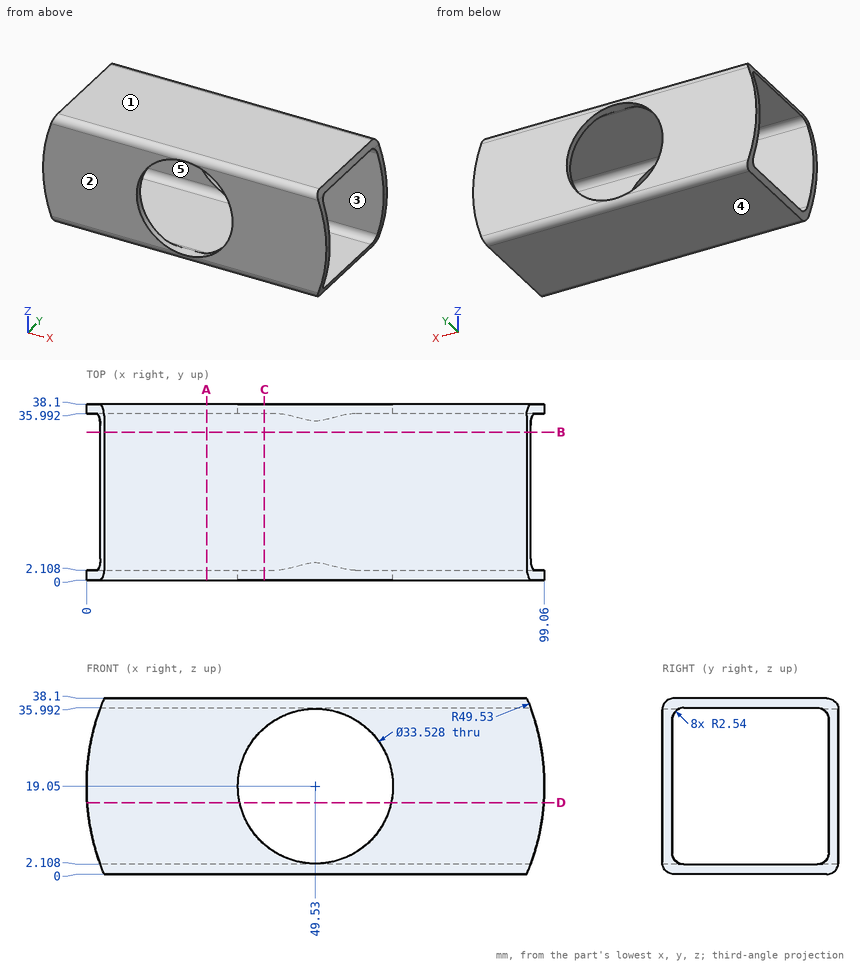
The drawing under review shows one solid part. Ordinate dimensions are in mm from its lowest x, y, z. A direction names the side the tool comes from. Give positions to 0.01 mm unless a question says otherwise; leave off trailing zeros. Write each loop counter-clockwise with the first axis right and the second up, starting at its lowest first coordinate (ties: lowest second). Pieces come first, ordered by that corner, then holes. Notation, with made-up numbers: M 83.5,57 L 125.5,57 A38 ccw 125.5,96 Z; hole C -34.75,69.25 d4. An arc over 180 degrees is marked long. Write each question's results on one line, items separated by ' | '. Start each with the question number.
1. We need section A-A (x = 26). Write out the cut boundary in (y, z).
2. Mouldability with a two-part tool opening along Y and no side actions: class the marked faces 1, 2 and 3 as released by +Y, released by -Y, zero draft, split by the parting line, or undercut.
3. We need section D-D (z = 15.5). Write out the cut boundary in (x, y).
4. For probe 1 along Y at (x, z) = (9, 7); probe 2 along Z at (x, y) = (49.53, 35.85), list the stretches that pass through material, from the lowest coordinate up. Write a range as [from, to].
5. For the marked faces 4 and 5, list the 3-axis set-ups (+Z, -Z, +X, -X, +Y, -Y) from which the entire face can be reached by the end or side of a thin tool; tool diameter is ignored.
6. We need section C-C (x = 38.5). Write out the cut boundary in (y, z), and give its area (3 significant figures).
7. We need section B-B (y = 32). Write out the cut boundary in (x, z), and give its area (3 significant figures).
8. Insertion check: pin 1 Ø12 at (y, z) = (34, 18.5) entering from -X. The pin has a flat end and moves straight along its axis. Give the tip position at first contact, or say it passes through.
Results found:
1) outline: M 0,2.54 A2.54 ccw 2.54,0 L 35.56,0 A2.54 ccw 38.1,2.54 L 38.1,35.56 A2.54 ccw 35.56,38.1 L 2.54,38.1 A2.54 ccw 0,35.56 Z; hole M 2.11,4.65 A2.54 ccw 4.65,2.11 L 33.45,2.11 A2.54 ccw 35.99,4.65 L 35.99,33.45 A2.54 ccw 33.45,35.99 L 4.65,35.99 A2.54 ccw 2.11,33.45 Z
2) face 1: zero draft | face 2: released by -Y | face 3: undercut
3) outline: M 0.13,0 L 33.15,0 L 33.15,2.11 L 0.13,2.11 Z; M 0.13,35.99 L 33.15,35.99 L 33.15,38.1 L 0.13,38.1 Z; M 65.91,0 L 98.93,0 L 98.93,2.11 L 65.91,2.11 Z; M 65.91,35.99 L 98.93,35.99 L 98.93,38.1 L 65.91,38.1 Z
4) probe 1: y = [0, 2.11], [35.99, 38.1] | probe 2: z = [0.02, 2.29], [35.81, 38.08]
5) face 4: -Z, +X, -X, +Y, -Y | face 5: +X, -X
6) outline: M 0,2.54 A2.54 ccw 2.54,0 L 35.56,0 A2.54 ccw 38.1,2.54 L 38.1,6.43 L 35.99,6.43 L 35.99,4.65 A2.54 cw 33.45,2.11 L 4.65,2.11 A2.54 cw 2.11,4.65 L 2.11,6.43 L 0,6.43 Z; M 0,31.67 L 2.11,31.67 L 2.11,33.45 A2.54 cw 4.65,35.99 L 33.45,35.99 A2.54 cw 35.99,33.45 L 35.99,31.67 L 38.1,31.67 L 38.1,35.56 A2.54 ccw 35.56,38.1 L 2.54,38.1 A2.54 ccw 0,35.56 Z | area: 197 mm^2
7) outline: M 2.99,2.11 A49.53 ccw 3.81,0 L 95.25,0 A49.53 ccw 96.07,2.11 Z; M 2.99,35.99 L 96.07,35.99 A49.53 ccw 95.25,38.1 L 3.81,38.1 A49.53 ccw Z | area: 389 mm^2
8) pin 1: stops at x = 0
